For this review, take the finished solid that the model builds, in its own axes (mm). Face numbers are marked on the shaded views. A direction names the side the tool comes from. Coordinates: 2 decimals unless noted, no trailing zeros. Write each loop counter-clockwise with the first axis right and the second up, starting at its lowest first coordinate (ties: lowest second). Pieces come first, ordered by that corner, then holes.
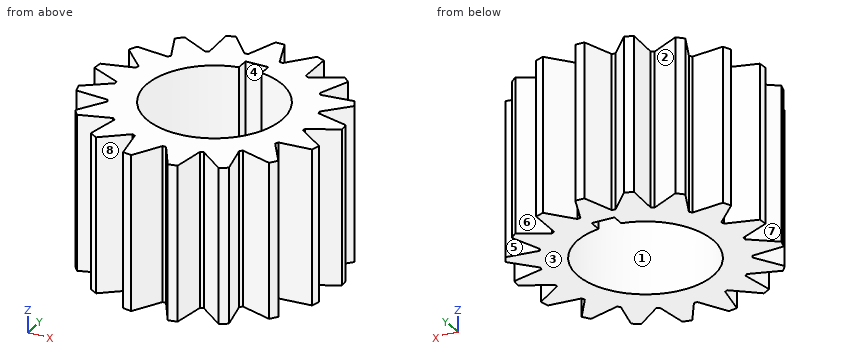
```python
from build123d import *

# Parameters (mm, degrees)
BOSS_EXTRUDE1_DEPTH = 43.5102
CUT_EXTRUDE1_DEPTH  = 43.5102


with BuildPart() as part:
    # Sketch2 → Boss-Extrude1 (new body)
    with BuildSketch(Plane.XY):
        with BuildLine():
            Line((-4.366026501, 25.941944541), (-1.27, 34.448207442))
            ThreePointArc((-1.27, 34.448207442), (0, 34.47161), (1.27, 34.448207442))
            Line((1.27, 34.448207442), (4.366026501, 25.941944541))
            ThreePointArc((4.366026501, 25.941944541), (4.83385814, 25.858857079), (5.300112805, 25.767333549))
            Line((5.300112805, 25.767333549), (11.259888122, 32.580773709))
            ThreePointArc((11.259888122, 32.580773709), (12.452581833, 32.143819028), (13.628367585, 31.663219877))
            Line((13.628367585, 31.663219877), (13.442509735, 22.612952173))
            ThreePointArc((13.442509735, 22.612952173), (13.848735094, 22.366475142), (14.250442508, 22.11270138))
            Line((14.250442508, 22.11270138), (22.26906596, 26.31312595))
            ThreePointArc((22.26906596, 26.31312595), (23.223373486, 25.474827181), (24.14614861, 24.601939015))
            Line((24.14614861, 24.601939015), (20.703507542, 16.229955312))
            ThreePointArc((20.703507542, 16.229955312), (20.993263634, 15.8533768), (21.276170986, 15.471626358))
            Line((21.276170986, 15.471626358), (30.270683044, 16.491744725))
            ThreePointArc((30.270683044, 16.491744725), (30.857719866, 15.365318762), (31.402858467, 14.218029965))
            Line((31.402858467, 14.218029965), (25.168381933, 7.655013053))
            ThreePointArc((25.168381933, 7.655013053), (25.302535593, 7.199192074), (25.428434676, 6.741022466))
            Line((25.428434676, 6.741022466), (34.184076646, 4.443061991))
            ThreePointArc((34.184076646, 4.443061991), (34.324560189, 3.180638903), (34.418438279, 1.913897183))
            Line((34.418438279, 1.913897183), (26.234126882, -1.953781138))
            ThreePointArc((26.234126882, -1.953781138), (26.194559914, -2.427283433), (26.14644736, -2.899993864))
            Line((26.14644736, -2.899993864), (33.480721277, -8.205680884))
            ThreePointArc((33.480721277, -8.205680884), (33.155678459, -9.433603865), (32.785617282, -10.648718018))
            Line((32.785617282, -10.648718018), (23.756807626, -11.298706359))
            ThreePointArc((23.756807626, -11.298706359), (23.54886377, -11.725940863), (23.333237446, -12.149349953))
            Line((23.333237446, -12.149349953), (28.255608976, -19.746201087))
            ThreePointArc((28.255608976, -19.746201087), (27.508938632, -20.773786158), (26.724917, -21.773164845))
            Line((26.724917, -21.773164845), (18.07099986, -19.117678678))
            ThreePointArc((18.07099986, -19.117678678), (17.722763084, -19.440945003), (17.36874452, -19.757869009))
            Line((17.36874452, -19.757869009), (19.214420114, -28.619887416))
            ThreePointArc((19.214420114, -28.619887416), (18.14696421, -29.308353518), (17.054868589, -29.95702511))
            Line((17.054868589, -29.95702511), (9.944603428, -24.354702557))
            ThreePointArc((9.944603428, -24.354702557), (9.503105039, -24.530341795), (9.058506404, -24.697978373))
            Line((9.058506404, -24.697978373), (7.578217344, -33.628299361))
            ThreePointArc((7.578217344, -33.628299361), (6.334141716, -33.884665333), (5.081465671, -34.095023136))
            Line((5.081465671, -34.095023136), (0.475133198, -26.302488901))
            ThreePointArc((0.475133198, -26.302488901), (0, -26.30678), (-0.475133198, -26.302488901))
            Line((-0.475133198, -26.302488901), (-5.081465671, -34.095023136))
            ThreePointArc((-5.081465671, -34.095023136), (-6.334141716, -33.884665333), (-7.578217344, -33.628299361))
            Line((-7.578217344, -33.628299361), (-9.058506404, -24.697978373))
            ThreePointArc((-9.058506404, -24.697978373), (-9.503105039, -24.530341795), (-9.944603428, -24.354702557))
            Line((-9.944603428, -24.354702557), (-17.054868589, -29.95702511))
            ThreePointArc((-17.054868589, -29.95702511), (-18.14696421, -29.308353518), (-19.214420114, -28.619887416))
            Line((-19.214420114, -28.619887416), (-17.36874452, -19.757869009))
            ThreePointArc((-17.36874452, -19.757869009), (-17.722763084, -19.440945003), (-18.07099986, -19.117678678))
            Line((-18.07099986, -19.117678678), (-26.724917, -21.773164845))
            ThreePointArc((-26.724917, -21.773164845), (-27.508938632, -20.773786158), (-28.255608976, -19.746201087))
            Line((-28.255608976, -19.746201087), (-23.333237446, -12.149349953))
            ThreePointArc((-23.333237446, -12.149349953), (-23.54886377, -11.725940863), (-23.756807626, -11.298706359))
            Line((-23.756807626, -11.298706359), (-32.785617282, -10.648718018))
            ThreePointArc((-32.785617282, -10.648718018), (-33.155678459, -9.433603865), (-33.480721277, -8.205680884))
            Line((-33.480721277, -8.205680884), (-26.14644736, -2.899993864))
            ThreePointArc((-26.14644736, -2.899993864), (-26.194559914, -2.427283433), (-26.234126882, -1.953781138))
            Line((-26.234126882, -1.953781138), (-34.418438279, 1.913897183))
            ThreePointArc((-34.418438279, 1.913897183), (-34.324560189, 3.180638903), (-34.184076646, 4.443061991))
            Line((-34.184076646, 4.443061991), (-25.428434676, 6.741022466))
            ThreePointArc((-25.428434676, 6.741022466), (-25.302535593, 7.199192074), (-25.168381933, 7.655013053))
            Line((-25.168381933, 7.655013053), (-31.402858467, 14.218029965))
            ThreePointArc((-31.402858467, 14.218029965), (-30.857719866, 15.365318762), (-30.270683044, 16.491744725))
            Line((-30.270683044, 16.491744725), (-21.276170986, 15.471626358))
            ThreePointArc((-21.276170986, 15.471626358), (-20.993263634, 15.8533768), (-20.703507542, 16.229955312))
            Line((-20.703507542, 16.229955312), (-24.14614861, 24.601939015))
            ThreePointArc((-24.14614861, 24.601939015), (-23.223373486, 25.474827181), (-22.26906596, 26.31312595))
            Line((-22.26906596, 26.31312595), (-14.250442508, 22.11270138))
            ThreePointArc((-14.250442508, 22.11270138), (-13.848735094, 22.366475142), (-13.442509735, 22.612952173))
            Line((-13.442509735, 22.612952173), (-13.628367585, 31.663219877))
            ThreePointArc((-13.628367585, 31.663219877), (-12.452581833, 32.143819028), (-11.259888122, 32.580773709))
            Line((-11.259888122, 32.580773709), (-5.300112805, 25.767333549))
            ThreePointArc((-5.300112805, 25.767333549), (-4.83385814, 25.858857079), (-4.366026501, 25.941944541))
        make_face()
    extrude(amount=BOSS_EXTRUDE1_DEPTH)

    # Sketch4 → Cut-Extrude1 (cut)
    with BuildSketch(Plane.XY.offset(43.5102)):
        with BuildLine():
            Line((-3.175, 22.225), (3.175, 22.225))
            Line((3.175, 22.225), (3.175, 18.783553311))
            ThreePointArc((3.175, 18.783553311), (0, -19.05), (-3.175, 18.783553311))
            Line((-3.175, 18.783553311), (-3.175, 22.225))
        make_face()
    extrude(amount=-CUT_EXTRUDE1_DEPTH, mode=Mode.SUBTRACT)


solid = part.part
```
1) Clearance check with flat-ended pins moving along their axes: P1, Ø4, axis at x = -7.5, y = -15, coming from the +Z side; P2, Ø3, axis at x = -24, z = 20, coming from the +Y side; P3, Ø4, axis at y = -12, z = 38.5, coming from the -X side; P4, Ø2, axis at y = -10.5, z = 23, coming from the +X side. State where each tip first meets the part, or that it passes through.
2) The part is to be moulded in two halves that separate along Y. For the marked faces 1, 2, 3 and 4, say which applies: pulls with the +Y half, pulls with the -Y half, needs draft (parallel to the pull), parting line crosses it, or undercut.
3) Consider section B-B (y = 0). Give the boundary of the cut face in (x, z).
4) For L1, parallel to Y at x = 0, z = 29.5 (3 decimals); L2, parallel to X at y = 30.5, z = 20.5; L3, parallel to X at y = 30, z = 21, list the stretches that pass through material, from the lowest coordinate up.
5) Tool access review of the marked faces 5, 6, 7 and 8: name each direction out of +Z, -Z, +X, -X, +Y, -Y from which nothing blocks a thin tool from reaching the whole face with its end or side.
6) Consider section A-A (y = 23.5). Give the boundary of the cut face in (x, z).
Results:
1. P1: passes through
1. P2: stops at y = 26.12
1. P3: stops at x = -32.99
1. P4: stops at x = 33.14
2. face 1: undercut
2. face 2: pulls with the +Y half
2. face 3: needs draft
2. face 4: undercut
3. outline: (-30.37, 0) - (-19.05, 0) - (-19.05, 43.51) - (-30.37, 43.51) - close; (19.05, 0) - (30.37, 0) - (30.37, 43.51) - (19.05, 43.51) - close
4. L1: y = -26.307 to -19.05, 22.225 to 34.472
4. L2: x = -13.6 to -9.44, -2.71 to 2.71, 9.44 to 13.6
4. L3: x = -13.59 to -9, -2.89 to 2.89, 9 to 13.59
5. face 5: +Z, -Z
5. face 6: +Z, -Z, +Y
5. face 7: +Z, -Z, -X
5. face 8: +Z, -Z, -Y
6. outline: (-23.69, 0) - (-16.9, 0) - (-16.9, 43.51) - (-23.69, 43.51) - close; (-13.46, 0) - (13.46, 0) - (13.46, 43.51) - (-13.46, 43.51) - close; (16.9, 0) - (23.69, 0) - (23.69, 43.51) - (16.9, 43.51) - close
